```python
from build123d import *

# Parameters (mm, degrees)
SKETCH1_R           = 6
BOSS_EXTRUDE1_DEPTH = 10
BOSS_EXTRUDE2_DEPTH = 3
CUT_EXTRUDE6_DEPTH  = 500


with BuildPart() as part:
    # Sketch1 → Boss-Extrude1 (new body)
    with BuildSketch(Plane(origin=(0, 0, 0), x_dir=(1, 0, 0), z_dir=(0, 1, 0))):
        with BuildLine():
            Line((0, 36), (48, 36))
            ThreePointArc((48, 36), (56.485281374, 32.485281374), (60, 24))
            Line((60, 24), (60, -24))
            ThreePointArc((60, -24), (56.485281374, -32.485281374), (48, -36))
            Line((48, -36), (-48, -36))
            ThreePointArc((-48, -36), (-56.485281374, -32.485281374), (-60, -24))
            Line((-60, -24), (-60, 24))
            ThreePointArc((-60, 24), (-56.485281374, 32.485281374), (-48, 36))
            Line((-48, 36), (0, 36))
        make_face()
        with Locations(Location((-48, 24, 0), (0, 0, 270))):
            Circle(SKETCH1_R, mode=Mode.SUBTRACT)
        with Locations(Location((48, 24, 0), (0, 0, 90))):
            Circle(SKETCH1_R, mode=Mode.SUBTRACT)
        with Locations(Location((48, -24, 0), (0, 0, 270))):
            Circle(SKETCH1_R, mode=Mode.SUBTRACT)
        with Locations(Location((-48, -24, 0), (0, 0, 90))):
            Circle(SKETCH1_R, mode=Mode.SUBTRACT)
    extrude(amount=BOSS_EXTRUDE1_DEPTH)

    # Sketch2 → Boss-Extrude2 (add)
    with BuildSketch(Plane(origin=(0, 10, 0), x_dir=(1, 0, 0), z_dir=(0, 1, 0))):
        Polygon((-25, 36), (-25, 11.04169411), (-25, -36), (25, -36), (25, 36), align=None)
    extrude(amount=BOSS_EXTRUDE2_DEPTH)

    # Sketch7 → Cut-Extrude6 (cut)
    with BuildSketch(Plane.XY.offset(36)):
        Polygon((-21.898641014, 3), (21.9, 3), (24.9, 0), (-25, 0), align=None)
    extrude(amount=-CUT_EXTRUDE6_DEPTH, mode=Mode.SUBTRACT)


solid = part.part
```
CAD build for the part. Positions are in the model's coordinates, mm. A direction names the side the tool comes from. Round coordinates to 2 decimals unless told otherwise and drop trailing zeros. Write each loop counter-clockwise with the first axis right and the second up, starting at its lowest first coordinate (ties: lowest second). Pieces come first, ordered by that corner, then holes. Notation, with made-up numbers: (53.5, -27.75) -> (105.5, -27.75) arc R27 ccw to (105.5, 10.25) -> close; hole circle Ø10 at (-16.75, -2.5). An arc over 180 degrees is marked (long way). Answer in a Markdown table with one row per item. Add a question column.
Item 1: Which spindle directions (+Z, -Z, +X, -X, +Y, -Y) get a long thin tool onto all of the face, cutting with end or side? Do faces 4 (the face through (-42, 0, -1)), 5 (the face through (0, 3, 1)), 6 (the face through (25, 11, 1)), 7 (the face through (60, 5, 0)), 8 (the face through (-42, 10, -1)). Say none if no direction does.
Item 2: Drop flat-ended pins along their axis: pin 1 Ø3.5 at (y, z) = (11.5, 13) entering from +X; pin 2 Ø6 at (x, z) = (-37.5, 17.5) entering from +Y; pin 3 Ø0.9 at (y, z) = (11, -11.5) entering from -X; pin 4 Ø9.5 at (x, z) = (-48, 24) entering from -Y. Give the stop position or say it passes through.
Item 3: Saw through at D-D, the plane x = 39.5. Write the cut outline in (y, z).
Item 4: Saw through at C-C, the plane y = 11.25. Write the cut outline in (x, z).
Item 5: Drill centre lines: line 1 (X direction, y = 6.5, z = -24); line 2 (X direction, y = 2.5, z = 24); line 3 (X direction, y = 9, z = -29). Where is each one in solid material? Low to high. Write a range as from..to.
Item 6: Saw through at A-A, the plane y = 4.25. Write the cut outline in (x, z).
Item 7: Mould opens along Z. For faces 1 (the face through (-48, 5, 30)), 2 (the face through (-60, 5, 0)), 3 (the face through (-1, 6, -36)) say: pulls with the +Z half, pulls with the -Z half, needs draft (parallel to the pull), parting line crosses it, or undercut.
Item 8: Saw through at B-B, the plane z = -21. Write the cut outline in (x, y), then the cut area to 3 significant figures.
Findings below:
| question | item | result |
|---|---|---|
| 1 | face 4 | +Z, -Z, +X, -X, -Y |
| 1 | face 5 | +Z, -Z, -Y |
| 1 | face 6 | +Z, -Z, +X, +Y |
| 1 | face 7 | +Z, -Z, +X, +Y, -Y |
| 1 | face 8 | +Z, -Z, -X, +Y |
| 2 | pin 1 | stops at x = 60 |
| 2 | pin 2 | stops at y = 10 |
| 2 | pin 3 | stops at x = -25 |
| 2 | pin 4 | passes through |
| 3 | outline | (0, -36) -> (10, -36) -> (10, 36) -> (0, 36) -> close |
| 4 | outline | (-25, -36) -> (25, -36) -> (25, 36) -> (-25, 36) -> close |
| 5 | line 1 | x = -60..-54, -42..42, 54..60 |
| 5 | line 2 | x = -60..-54, -42..-22.42, 22.4..42, 54..60 |
| 5 | line 3 | x = -58.91..-51.32, -44.68..44.68, 51.32..58.91 |
| 6 | outline | (-60, -24) arc R12 ccw to (-48, -36) -> (48, -36) arc R12 ccw to (60, -24) -> (60, 24) arc R12 ccw to (48, 36) -> (-48, 36) arc R12 ccw to (-60, 24) -> close; hole circle Ø12 at (-48, -24); hole circle Ø12 at (-48, 24); hole circle Ø12 at (48, -24); hole circle Ø12 at (48, 24) |
| 7 | face 1 | undercut |
| 7 | face 2 | needs draft |
| 7 | face 3 | pulls with the -Z half |
| 8 | outline | (-60, 0) -> (-53.2, 0) -> (-53.2, 10) -> (-60, 10) -> close; (-42.8, 0) -> (-25, 0) -> (-21.9, 3) -> (21.9, 3) -> (24.9, 0) -> (42.8, 0) -> (42.8, 10) -> (25, 10) -> (25, 13) -> (-25, 13) -> (-25, 10) -> (-42.8, 10) -> close; (53.2, 0) -> (60, 0) -> (60, 10) -> (53.2, 10) -> close |
| 8 | area | 1,000 mm^2 |
